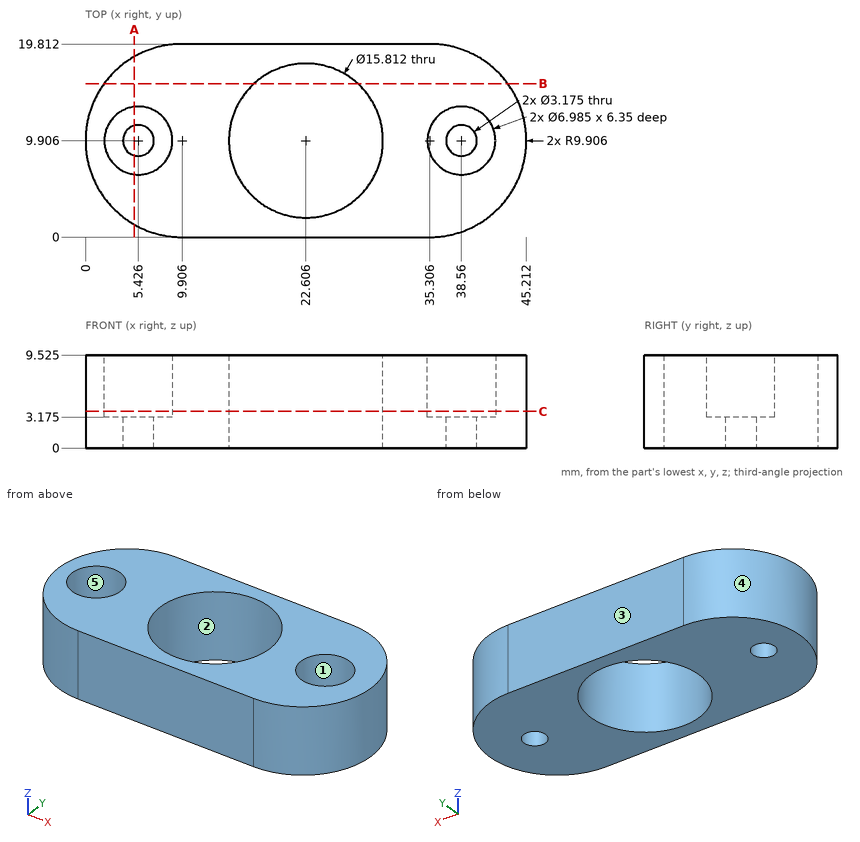
Part print with two shaded views. Sizes in mm from the minimum x, y, z corner. A direction names the side the tool comes from. Round coordinates to 2 decimals unless told otherwise and drop trailing zeros. Order: outer loops, then holes, each group sorted by start corner. A loop starts at its lowest first (then second) coordinate and runs counter-clockwise, first axis right, second up. Notation, with made-up numbers: M 30.25,14.5 L 34.25,14.5 A15 ccw 34.25,42.5 Z; hole C 18.25,22.25 d4. An arc over 180 degrees is marked long. Use CSV: the item, a comma, the result in double quotes.
Item 1: Saw through at C-C (z = 3.75). List the corners of the cut face in (x, y) (1 decimal).
Worked answers:
outline,"M 9.9,0 L 35.3,0 A9.9 ccw 35.3,19.8 L 9.9,19.8 A9.9 ccw Z; hole C 5.4,9.9 d7; hole C 22.6,9.9 d15.8; hole C 38.6,9.9 d7"
Item 2: Pin check, flat tips, straight feed: pin 1 (5.5 mm diameter, centred on x = 39, y = 11, fed in from +Z) (1 decimal); pin 2 (2 mm diameter, centred on y = 2, z = 5.5, fed in from +X); pin 3 (1 mm diameter, centred on y = 5.5, z = 7.5, fed in from +X); pin 4 (5 mm diameter, centred on y = 2, z = 6, fed in from +X). Stop position of each tip, or through.
Worked answers:
pin 1,"z = 9.5"
pin 2,"x = 42.41"
pin 3,"x = 44.41"
pin 4,"x = 43.61"
Item 3: Which spindle directions (+Z, -Z, +X, -X, +Y, -Y) get a long thin tool onto all of the face, cutting with end or side? Do the marked faces 1 and 2. Say none if no direction does.
Worked answers:
face 1,"+Z"
face 2,"+Z, -Z"
Item 4: Pull direction Y, two halves, no side cores. Call the marked faces 3, 4 and 5: released by +Y, released by -Y, zero draft, split by the parting line, or undercut.
Worked answers:
face 3,"released by +Y"
face 4,"split by the parting line"
face 5,"undercut"
Item 5: Saw through at A-A (x = 5). List the corners of the cut face in (y, z) (1 decimal).
Worked answers:
outline,"M 1.3,0 L 8.4,0 L 8.4,3.2 L 6.4,3.2 L 6.4,9.5 L 1.3,9.5 Z; M 11.4,0 L 18.5,0 L 18.5,9.5 L 13.4,9.5 L 13.4,3.2 L 11.4,3.2 Z"
Item 6: Probe probe 1 along X at (y, z) = (7.5, 8.5) (1 decimal); probe 2 along X at (y, z) = (9, 9.25); probe 3 along Y at (x, z) = (22.5, 9.25). List the from-to ranges inside material, lowest first.
Worked answers:
probe 1,"0.3 to 2.9, 8 to 15.1, 30.1 to 36, 41.1 to 44.9"
probe 2,"0.04 to 2.05, 8.8 to 14.75, 30.46 to 35.19, 41.93 to 45.17"
probe 3,"0 to 2, 17.81 to 19.81"
Item 7: Saw through at B-B (y = 15.75). List the corners of the cut face in (x, z) (1 decimal).
Worked answers:
outline,"M 1.9,0 L 17.3,0 L 17.3,9.5 L 1.9,9.5 Z; M 27.9,0 L 43.3,0 L 43.3,9.5 L 27.9,9.5 Z"
